Could you check a few things on this drawing? It's one solid part, dimensions in mm from its lowest x, y, z. A direction names the side the tool comes from. Give positions to 0.01 mm unless a question says otherwise; leave off trailing zeros. Loops run counter-clockwise (first coordinate to the right, second up) from the corner with the lowest first, then second, coordinate; pieces in that order, holes last. Notation, with made-up numbers: (65.25, 68) - (93.25, 68) arc R16 ccw to (93.25, 85) - close; hole circle Ø10 at (38.5, 21). An arc over 180 degrees is marked (long way). Return JSON: item names as keys, results as strings. Group by question number.
(1) For P1, Ø2, axis at y = 26.5, z = 39, coming from the +X side; P2, Ø10, axis at x = 31.5, z = 33, coming from the +Y side; P3, Ø5, axis at x = 5.5, y = 4, coming from the +Z side, each with a flat end and sliding along its axis, tell me the tip position at first contact or that it passes through.
(2) If we section it at D-D (x = 24.5): Please give me the cut outline in (y, z), then the cut area to 3 significant figures.
(3) I need wall thicknesses on probe 1 along X at (y, z) = (5, 29.5); probe 2 along X at (y, z) = (27.5, 42); probe 3 along X at (y, z) = (27, 23). Which ranges of each line are inside material? Lowest first, please. Write a range as [from, to].
(4) On a 3-axis mill with a long thin cutter (end or side, diameter ignored), from which of +Z, -Z, +X, -X, +Y, -Y can I reach the whole of each face in a straight line? I mean the marked faces 1, 2 and 3. Say none if no direction works.
(5) If we section it at B-B (y = 8.5): Please give me the cut outline in (x, z), then the cut area to 3 significant figures.
(6) If we section it at A-A (x = 5): Please give me the cut outline in (y, z), then the cut area to 3 significant figures.
(7) If we mould it in two halves opening along Z, with no side actions, what happens to the marked faces 4, 5 and 6? For each: released by +Z, released by -Z, zero draft, split by the parting line, or undercut.
(8) If we section it at C-C (z = 14.5): Please give me the cut outline in (x, y), then the cut area to 3 significant figures.
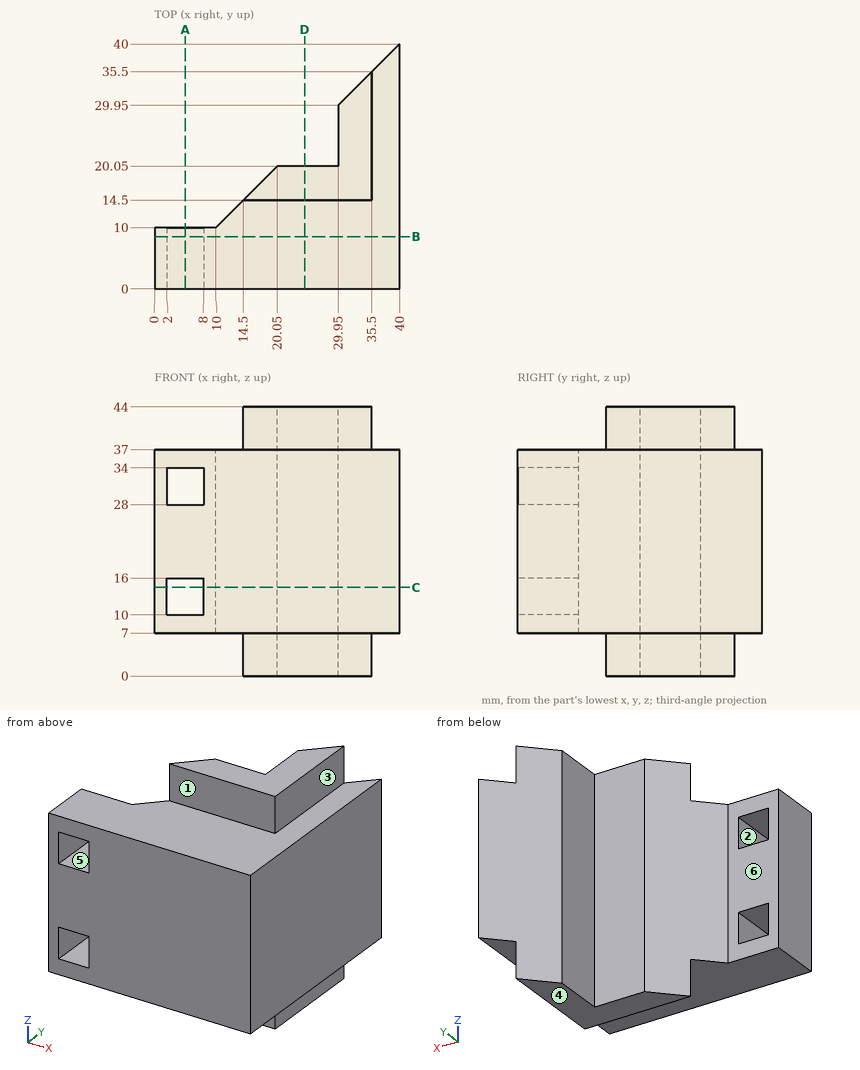
Values:
{
 "1": {"P1": "x = 35.5", "P2": "y = 36.5", "P3": "z = 37"},
 "2": {"outline": "(0, 7) - (14.5, 7) - (14.5, 0) - (20.05, 0) - (20.05, 44) - (14.5, 44) - (14.5, 37) - (0, 37) - close", "area": "679 mm2"},
 "3": {"probe 1": "[0, 2], [8, 40]", "probe 2": "[29.95, 35.5]", "probe 3": "[29.95, 40]"},
 "4": {"face 1": "+Z, +X, -X, -Y", "face 2": "+Y, -Y", "face 3": "+Z, +X, +Y, -Y"},
 "5": {"outline": "(0, 7) - (40, 7) - (40, 37) - (0, 37) - close; hole (2, 10) - (8, 10) - (8, 16) - (2, 16) - close; hole (2, 28) - (8, 28) - (8, 34) - (2, 34) - close", "area": "1,130 mm2"},
 "6": {"outline": "(0, 7) - (10, 7) - (10, 10) - (0, 10) - close; (0, 16) - (10, 16) - (10, 28) - (0, 28) - close; (0, 34) - (10, 34) - (10, 37) - (0, 37) - close", "area": "180 mm2"},
 "7": {"face 4": "released by -Z", "face 5": "undercut", "face 6": "zero draft"},
 "8": {"outline": "(0, 0) - (2, 0) - (2, 10) - (0, 10) - close; (8, 0) - (40, 0) - (40, 40) - (29.95, 29.95) - (29.95, 20.05) - (20.05, 20.05) - (10, 10) - (8, 10) - close", "area": "741 mm2"}
}
